The listing builds one solid part. Answer for the finished solid, in the listing's coordinates (mm). Face numbers are marked on the shaded views. A direction names the side the tool comes from. Coordinates: 2 decimals unless noted, no trailing zeros. Loops run counter-clockwise (first coordinate to the right, second up) from the corner with the lowest first, then second, coordinate; pieces in that order, holes last. Notation, with made-up numbers: M 30,27.5 L 40,27.5 A19 ccw 40,63.5 Z; hole C 33.25,27 d1. An arc over 180 degrees is marked long. Answer as a JSON object with one key per item and string values. Group by question number.
1. A cutting plane is placed at D-D on x = -5. State how many separate pieces and enclosed holes the cut face has, and give its area (3 significant figures).
2. A cutting plane is placed at C-C on x = 8. Give the vertices of the cut face in (y, z), and give its area (3 significant figures).
3. A cutting plane is placed at B-B on z = 1.25. Give the vertices of the cut face in (x, y), and give its area (3 significant figures).
4. Straight lines are drawn through the part: L1, parallel to Y at x = -5, z = 9.65 (3 decimals); L2, parallel to Z at x = -2.5, y = 25. For each, find the intervals that lie inside material, in ascending order.
5. Determine the mould class of the marked faces 1, 2 and 3 for opening direction Z: released by +Z, released by -Z, zero draft, split by the parting line, or undercut.
6. For the marked faces 4 and 5, determine the directions among +Z, -Z, +X, -X, +Y, -Y from which every point of the face is accessible in a straight line to the end or side of a thin tool.
7. A cutting plane is placed at A-A on y = 32.5. Give the vertices of the cut face in (x, z), and give its area (3 significant figures).
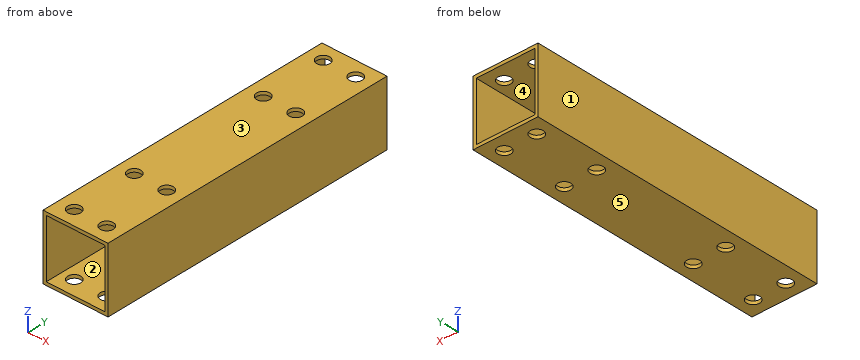
from build123d import *

# Parameters (mm, degrees)
SKETCH_1_W          = 20
SKETCH_1_H          = 20
SKETCH_1_W_2        = 18
SKETCH_1_H_2        = 18
EXTRUDE_1_DEPTH     = 93
SKETCH_2_R          = 2.025
CUT_EXTRUDE_1_DEPTH = 21


with BuildPart() as part:
    # 草图1 → 凸台-拉伸1 (new body)
    with BuildSketch(Plane(origin=(0, 0, 0), x_dir=(1, 0, 0), z_dir=(0, 1, 0))):
        Rectangle(SKETCH_1_W, SKETCH_1_H)
        Rectangle(SKETCH_1_W_2, SKETCH_1_H_2, mode=Mode.SUBTRACT)
    extrude(amount=EXTRUDE_1_DEPTH)

    # 草图2 → 切除-拉伸1 (cut, through all)
    with BuildSketch(Plane.XY.offset(10)):
        with Locations((-5, 5)):
            Circle(SKETCH_2_R)
        with Locations((-5, 25)):
            Circle(SKETCH_2_R)
        with Locations((5, 25)):
            Circle(SKETCH_2_R)
        with Locations((5, 5)):
            Circle(SKETCH_2_R)
        with Locations((5, 88)):
            Circle(SKETCH_2_R)
        with Locations((-5, 88)):
            Circle(SKETCH_2_R)
        with Locations((-5, 68)):
            Circle(SKETCH_2_R)
        with Locations((5, 68)):
            Circle(SKETCH_2_R)
    extrude(amount=-CUT_EXTRUDE_1_DEPTH, mode=Mode.SUBTRACT)


solid = part.part
From the geometry:
{
 "1": {"separate pieces": "10", "enclosed holes": "0", "area": "154 mm²"},
 "2": {"outline": "M 0,-10 L 93,-10 L 93,-9 L 0,-9 Z; M 0,9 L 93,9 L 93,10 L 0,10 Z", "area": "186 mm²"},
 "3": {"outline": "M -10,0 L -9,0 L -9,93 L -10,93 Z; M 9,0 L 10,0 L 10,93 L 9,93 Z", "area": "186 mm²"},
 "4": {"L1": "y = 0 to 2.975, 7.025 to 22.975, 27.025 to 65.975, 70.025 to 85.975, 90.025 to 93", "L2": "z = -10 to -9, 9 to 10"},
 "5": {"face 1": "zero draft", "face 2": "undercut", "face 3": "released by +Z"},
 "6": {"face 4": "+Y, -Y", "face 5": "-Z, +X, -X, +Y, -Y"},
 "7": {"outline": "M -10,-10 L 10,-10 L 10,10 L -10,10 Z; hole M -9,-9 L 9,-9 L 9,9 L -9,9 Z", "area": "76.0 mm²"}
}
